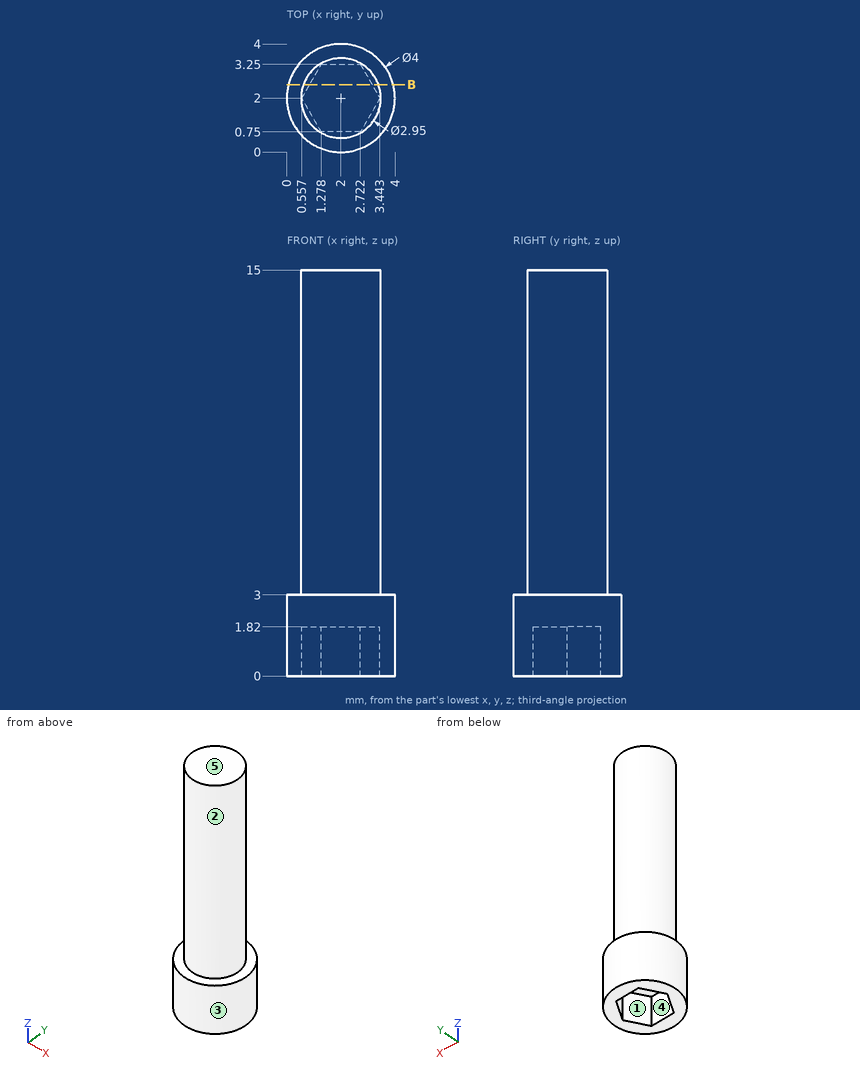
The figure shows three views and two pictorial views of one solid part (mm, origin at its lowest corner). Answer the questions. A direction names the side the tool comes from. Round coordinates to 2 decimals unless told otherwise and drop trailing zeros. Write each loop counter-clockwise with the first axis right and the second up, starting at its lowest first coordinate (ties: lowest second). Pieces come first, ordered by that corner, then holes. Notation, with made-up numbers: (67, 22) - (72, 22) arc R24 ccw to (72, 38) - close; hole circle Ø3 at (-31, 58.25). An arc over 180 degrees is marked (long way). One line per question, with ' | ' between items. Start each with the question number.
1. Section B-B (y = 2.5) is taken. Determine the outline of the cut face in (x, z) (1 decimal).
2. For a pull along Y with two mould halves and no side action, classify the marked faces 3, 4 and 5 as +Y half, -Y half, draft (parallel to the pull), parting line (faces both ways), or undercut.
3. For the marked faces 1 and 2, determine the directions among +Z, -Z, +X, -X, +Y, -Y from which every point of the face is accessible in a straight line to the end or side of a thin tool.
4. Find the intervals of material crossed by probe 1 along Z at (x, y) = (1.25, 3.8); probe 2 along Z at (x, y) = (2.4, 2.2); probe 3 along Y at (x, z) = (3.15, 1.25) (1 decimal), in increasing order. Write a range as [from, to].
Filled in:
1) outline: (0.1, 0) - (0.8, 0) - (0.8, 1.8) - (3.2, 1.8) - (3.2, 0) - (3.9, 0) - (3.9, 3) - (3.4, 3) - (3.4, 15) - (0.6, 15) - (0.6, 3) - (0.1, 3) - close
2) face 3: parting line | face 4: undercut | face 5: draft
3) face 1: -Z | face 2: +Z
4) probe 1: [0, 3] | probe 2: [1.82, 15] | probe 3: [0.4, 1.5], [2.5, 3.6]
